Could you check a few things on this drawing? It's one solid part, dimensions in mm from its lowest x, y, z. A direction names the side the tool comes from. Coordinates: 2 decimals unless noted, no trailing zeros. Order: outer loops, then holes, each group sorted by start corner. A loop starts at its lowest first (then second) coordinate and runs counter-clockwise, first axis right, second up.
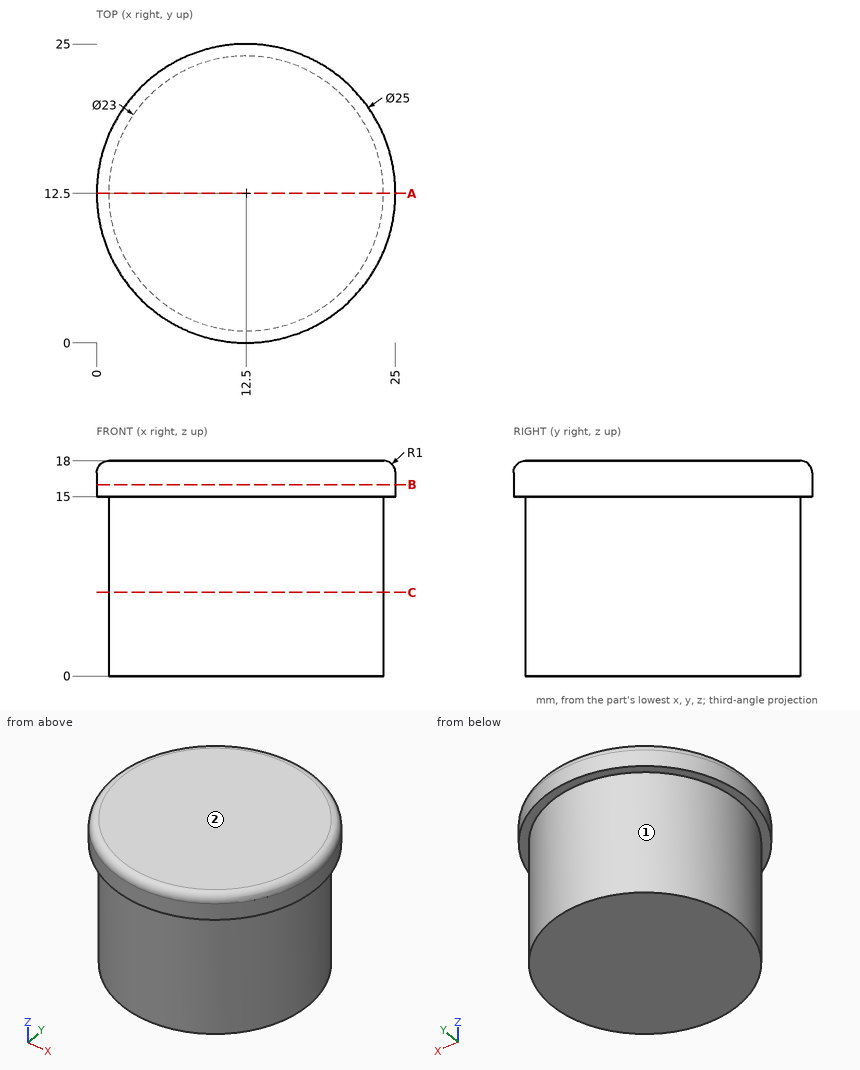
1. Imagine slicing it at A-A on y = 12.5. Please give me the cut outline in (x, z), then the cut area to 3 significant figures.
Completed:
outline: (0, 15) - (1, 15) - (1, 0) - (24, 0) - (24, 15) - (25, 15) - (25, 17) arc R1 ccw to (24, 18) - (1, 18) arc R1 ccw to (0, 17) - close
area: 420 mm2
2. I'm going to push flat-ended pins straight in: pin 1 (8 mm diameter, centred on x = 12.5, z = 8, fed in from -Y); pin 2 (8 mm diameter, centred on x = 15.5, z = 12, fed in from -Y) (3 decimals); pin 3 (5 mm diameter, centred on x = 16.5, z = 3, fed in from +Y). Where does each tip first touch, or does it pass through?
Completed:
pin 1: stops at y = 1
pin 2: stops at y = 0.005
pin 3: stops at y = 23.9
3. Imagine slicing it at B-B on z = 16. Please give me the cut outline in (x, y).
Completed:
outline: circle Ø25 at (12.5, 12.5)
4. Imagine slicing it at C-C on z = 7. Please give me the cut outline in (x, y).
Completed:
outline: circle Ø23 at (12.5, 12.5)
5. On a 3-axis mill with a long thin cutter (end or side, diameter ignored), from which of +Z, -Z, +X, -X, +Y, -Y can I reach the whole of each face in a straight line? I mean the marked faces 1 and 2. Say none if no direction works.
Completed:
face 1: -Z
face 2: +Z, +X, -X, +Y, -Y
6. Please list where these lines run through material, in increasing order: probe 1 along Y at (x, z) = (4.75, 1.25); probe 2 along X at (y, z) = (5.5, 3.25); probe 3 along Y at (x, z) = (17.25, 15.5).
Completed:
probe 1: y = 4 to 21
probe 2: x = 3.38 to 21.62
probe 3: y = 0.94 to 24.06
